```python
from build123d import *

# Parameters (mm, degrees)
BOSS_EXTRUDE1_DEPTH = 4
SKETCH5_R           = 1.5
CUT_EXTRUDE1_DEPTH  = 3
SKETCH6_R           = 1.5
CUT_EXTRUDE2_DEPTH  = 3
FILLET1_R           = 2
FILLET2_R           = 1


with BuildPart() as part:
    # Sketch4 → Boss-Extrude1 (new body)
    with BuildSketch(Plane(origin=(0, 0, 0), x_dir=(0, 1, 0), z_dir=(0, 0, 1))):
        with BuildLine():
            Line((-2, -27.920633468), (-2, -39.763932023))
            ThreePointArc((-2, -39.763932023), (0, -45), (2, -39.763932023))
            Line((2, -39.763932023), (2, -27.920633468))
            Line((2, -27.920633468), (4.867831403, -20.764056013))
            Line((4.867831403, -20.764056013), (4.867831403, -14.872797682))
            Line((4.867831403, -14.872797682), (12.044370558, -14.872797682))
            Line((12.044370558, -14.872797682), (34.004647608, -36.833074732))
            ThreePointArc((34.004647608, -36.833074732), (39.121320344, -39.121320344), (36.833074732, -34.004647608))
            Line((36.833074732, -34.004647608), (17.701224807, -14.872797682))
            Line((17.701224807, -14.872797682), (22.894335258, -14.872797682))
            Line((22.894335258, -14.872797682), (28.248854336, -9.518278604))
            Line((28.248854336, -9.518278604), (28.248854336, 24.78907846))
            Line((28.248854336, 24.78907846), (38.365899309, 34.906123433))
            Line((38.365899309, 34.906123433), (39.093876567, 35.634100691))
            ThreePointArc((39.093876567, 35.634100691), (37.77325109, 39.377410935), (34.503238183, 37.127202318))
            Line((34.503238183, 37.127202318), (24.284388241, 37.127202318))
            Line((24.284388241, 37.127202318), (19.784388241, 41.627202318))
            Line((19.784388241, 41.627202318), (2.472048116, 41.627202318))
            ThreePointArc((2.472048116, 41.627202318), (0, 44.5), (-2.472048116, 41.627202318))
            Line((-2.472048116, 41.627202318), (-10.570956119, 41.627202318))
            Line((-10.570956119, 41.627202318), (-10.570956119, -14.872797682))
            Line((-10.570956119, -14.872797682), (-4.867831403, -14.872797682))
            Line((-4.867831403, -14.872797682), (-4.867831403, -20.764056013))
            Line((-4.867831403, -20.764056013), (-2, -27.920633468))
        make_face()
        with BuildLine():
            ThreePointArc((-2.867831403, -20.065196532), (0, -17.197365128), (2.867831403, -20.065196532))
            Line((2.867831403, -20.065196532), (2.867831403, -21.860808403))
            ThreePointArc((2.867831403, -21.860808403), (0, -24.728639806), (-2.867831403, -21.860808403))
            Line((-2.867831403, -21.860808403), (-2.867831403, -20.065196532))
        make_face(mode=Mode.SUBTRACT)
        with BuildLine():
            Line((15.992780239, -12.872797682), (-8.570956119, -12.872797682))
            Line((-8.570956119, -12.872797682), (-8.570956119, 5.127202318))
            Line((-8.570956119, 5.127202318), (-4.107420483, 5.127202318))
            Line((-4.107420483, 5.127202318), (-4.107420483, 20.127202318))
            Line((-4.107420483, 20.127202318), (-8.570956119, 20.127202318))
            Line((-8.570956119, 20.127202318), (-8.570956119, 39.627202318))
            Line((-8.570956119, 39.627202318), (14.71332043, 39.627202318))
            Line((14.71332043, 39.627202318), (18.481087383, 35.859435365))
            ThreePointArc((18.481087383, 35.859435365), (19.292145755, 35.317503486), (20.248854336, 35.127202318))
            Line((20.248854336, 35.127202318), (26.248854336, 35.127202318))
            Line((26.248854336, 35.127202318), (26.248854336, -4.702478507))
            Line((26.248854336, -4.702478507), (26.248854336, -8.550773098))
            Line((26.248854336, -8.550773098), (15.992780239, -8.550773098))
            Line((15.992780239, -8.550773098), (15.992780239, -12.872797682))
        make_face(mode=Mode.SUBTRACT)
        Polygon((34.905300686, 34.273951935), (28.248854336, 27.617505584), (28.248854336, 35.127202318), (34.905300686, 35.127202318), align=None, mode=Mode.SUBTRACT)
    extrude(amount=BOSS_EXTRUDE1_DEPTH)

    # Sketch5 → Cut-Extrude1 (cut)
    with BuildSketch(Plane.XY.offset(4)):
        with Locations((-37, 37)):
            Circle(SKETCH5_R)
        with Locations((-42, 0)):
            Circle(SKETCH5_R)
        with Locations((37, 37)):
            Circle(SKETCH5_R)
        with Locations((42, 0)):
            Circle(SKETCH5_R)
    extrude(amount=-CUT_EXTRUDE1_DEPTH, mode=Mode.SUBTRACT)

    # Sketch6 → Cut-Extrude2 (cut)
    with BuildSketch(Plane(origin=(0, 0, 0), x_dir=(1, 0, 0), z_dir=(0, 0, -1))):
        with Locations(Location((-17.127202318, 7.251145664, 0), (0, 0, 180))):
            Circle(SKETCH6_R)
        with Locations(Location((-9.127202318, 7.251145664, 0), (0, 0, 180))):
            Circle(SKETCH6_R)
        with Locations(Location((11.372797682, -20.248854336, 0), (0, 0, 180))):
            Circle(SKETCH6_R)
        with Locations(Location((-37.627202318, -20.248854336, 0), (0, 0, 180))):
            Circle(SKETCH6_R)
    extrude(amount=-CUT_EXTRUDE2_DEPTH, mode=Mode.SUBTRACT)

    # Fillet1
    fillet1_edges = [part.edges().sort_by_distance(p)[0] for p in [
        (-41.627202318, 19.784388241, 2),
        (-37.127202318, 24.284388241, 2),
        (-37.127202318, 34.503238183, 2),
        (-24.78907846, 28.248854336, 2),
        (9.518278604, 28.248854336, 2),
        (14.872797682, 22.894335258, 2),
        (34.004647608, 36.833074732, 2),
        (36.833074732, 34.004647608, 2),
        (14.872797682, 12.044370558, 2),
        (14.872797682, 4.867831403, 2),
        (20.764056013, 4.867831403, 2),
        (27.920633468, 2, 2),
        (39.763932023, 2, 2),
        (39.763932023, -2, 2),
        (27.920633468, -2, 2),
        (20.764056013, -4.867831403, 2),
        (14.872797682, -4.867831403, 2),
        (14.872797682, -10.570956119, 2),
        (-41.627202318, -10.570956119, 2),
        (-41.627202318, -2.472048116, 2),
        (-41.627202318, 2.472048116, 2),
        (-39.627202318, 14.71332043, 2),
        (-20.127202318, -4.107420483, 2),
        (-5.127202318, -4.107420483, 2),
        (12.872797682, 15.992780239, 2),
        (8.550773098, 15.992780239, 2),
        (8.550773098, 26.248854336, 2),
    ]]
    fillet(fillet1_edges, radius=FILLET1_R)

    # Fillet2
    # the kernel refuses this fillet: 1 mm, written as the material it adds along each edge
    with BuildSketch(Plane(origin=(14.872797682, 17.701224807, 0), x_dir=(0, 1, 0), z_dir=(0, 0, 1))) as fillet2_piece_1:
        with BuildLine():
            CenterArc((FILLET2_R * 2.41421356237, -FILLET2_R), FILLET2_R, 90, 135)
            Line((FILLET2_R * 1.70710678119, -FILLET2_R * 1.70710678119), (0, 0))
            Line((0, 0), (FILLET2_R * 2.41421356237, 0))
        make_face()
    extrude(amount=4)
    with BuildSketch(Plane(origin=(-34.273951935, 34.905300686, 0), x_dir=(0.7071067811865476, -0.7071067811865476, 0), z_dir=(0, 0, 1))) as fillet2_piece_2:
        with BuildLine():
            CenterArc((FILLET2_R * 0.414213562373, -FILLET2_R), FILLET2_R, 90, 45)
            Line((-FILLET2_R * 0.292893218813, -FILLET2_R * 0.292893218814), (0, 0))
            Line((0, 0), (FILLET2_R * 0.414213562373, 0))
        make_face()
    extrude(amount=4)
    with BuildSketch(Plane(origin=(-35.127202318, 34.905300686, 0), x_dir=(1, 0, 0), z_dir=(0, 0, 1))) as fillet2_piece_3:
        with BuildLine():
            CenterArc((FILLET2_R, -FILLET2_R), FILLET2_R, 90, 90)
            Line((0, -FILLET2_R), (0, 0))
            Line((0, 0), (FILLET2_R, 0))
        make_face()
    extrude(amount=4)
    with BuildSketch(Plane(origin=(-35.127202318, 28.248854336, 0), x_dir=(1, 0, 0), z_dir=(0, 0, 1))) as fillet2_piece_4:
        with BuildLine():
            CenterArc((FILLET2_R, FILLET2_R), FILLET2_R, 180, 90)
            Line((0, FILLET2_R), (0, 0))
            Line((0, 0), (FILLET2_R, 0))
        make_face()
    extrude(amount=4)
    with BuildSketch(Plane(origin=(-27.617505584, 28.248854336, 0), x_dir=(-0.7071067811865468, 0.7071067811865482, 0), z_dir=(0, 0, 1))) as fillet2_piece_5:
        with BuildLine():
            CenterArc((FILLET2_R * 2.41421356237, FILLET2_R), FILLET2_R, 135, 135)
            Line((FILLET2_R * 1.70710678119, FILLET2_R * 1.70710678119), (0, 0))
            Line((0, 0), (FILLET2_R * 2.41421356237, 0))
        make_face()
    extrude(amount=4)


solid = part.part
```
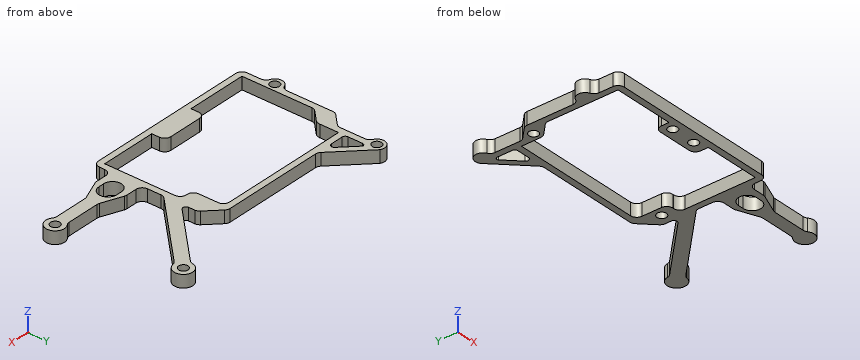
Check sheet for the modelled part. Datum: model origin and axes. Units: mm. Coordinates: 2 decimals unless noted, no trailing zeros. Write each loop counter-clockwise with the first axis right and the second up, starting at its lowest first coordinate (ties: lowest second). Pieces come first, ordered by that corner, then holes. Notation, with made-up numbers: (82.25, 41) -> (136.25, 41) arc R20 ccw to (136.25, 51) -> close; hole circle Ø2 at (28, 0). An arc over 180 degrees is marked (long way). Use a Markdown table: item, result.
1. Go/stop test with flat-tipped pins: pin 1 Ø2 at (x, z) = (33.5, 1) entering from +Y; pin 2 Ø1.5 at (y, z) = (28, 1) entering from -X; pin 3 Ø1.5 at (x, y) = (-41.5, 0.5) entering from +Z. Record where each tip stops, or that it passes through.
Reported:
| item | result |
|---|---|
| pin 1 | stops at y = 38.66 |
| pin 2 | stops at x = -37.13 |
| pin 3 | stops at z = 1 |
2. Sectioned sample at D-D (x = 31). Enter the section's corners in (y, z), plus the area to 3 significant figures.
Reported:
| item | result |
|---|---|
| outline | (-2, 0) -> (2, 0) -> (2, 4) -> (-2, 4) -> close; (28.17, 0) -> (33.83, 0) -> (33.83, 4) -> (28.17, 4) -> close |
| area | 38.6 mm2 |
3. Scan lines: line 1 along Y through (x, z) = (6, 1.8); line 2 along Y through (x, z) = (-38, 3.1); line 3 along Y through (x, z) = (-33.5, 1.55). Record each from-to range of solid material in increasing order.
Reported:
| item | result |
|---|---|
| line 1 | y = -10.57 to -8.57, 26.25 to 28.25 |
| line 2 | y = -10.57 to -8.57, 16.34 to 23.41, 34.69 to 35.88, 38.12 to 39.29 |
| line 3 | y = -10.57 to -8.57, 26.25 to 28.25, 34.13 to 36.96 |
4. Sectioned sample at C-C (z = 2.1). Give the number of separate pieces and of enclosed holes in the cut face, plus the area to 3 significant figures.
Reported:
| item | result |
|---|---|
| separate pieces | 1 |
| enclosed holes | 11 |
| area | 778 mm2 |
5. Sectioned sample at A-A (y = 0). Enter the section's corners in (x, z), plus the area to 3 significant figures.
Reported:
| item | result |
|---|---|
| outline | (-44.5, 0) -> (-39.63, 0) -> (-39.63, 4) -> (-40.5, 4) -> (-40.5, 1) -> (-43.5, 1) -> (-43.5, 4) -> (-44.5, 4) -> close; (12.87, 0) -> (17.2, 0) -> (17.2, 4) -> (12.87, 4) -> close; (24.73, 0) -> (45, 0) -> (45, 4) -> (43.5, 4) -> (43.5, 1) -> (40.5, 1) -> (40.5, 4) -> (24.73, 4) -> close |
| area | 99.9 mm2 |
6. Sectioned sample at B-B (x = 4). Enter the section's corners in (y, z).
Reported:
| item | result |
|---|---|
| outline | (-10.57, 0) -> (-8.57, 0) -> (-8.57, 4) -> (-10.57, 4) -> close; (26.25, 0) -> (28.25, 0) -> (28.25, 4) -> (26.25, 4) -> close |
